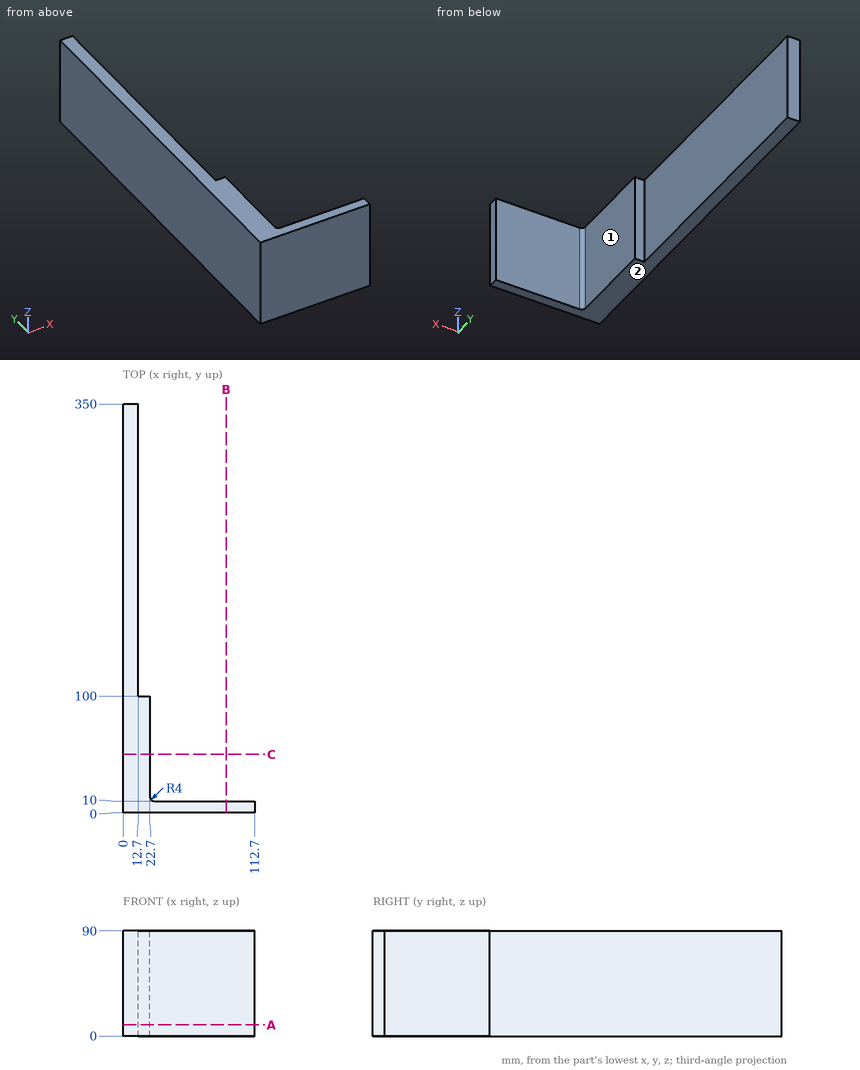
The figure shows three views and two pictorial views of one solid part (mm, origin at its lowest corner). Answer the questions. A direction names the side the tool comes from. Give positions to 0.01 mm unless a question says otherwise; leave off trailing zeros. Order: outer loops, then holes, each group sorted by start corner. A loop starts at its lowest first (then second) coordinate and runs counter-clockwise, first axis right, second up. Notation, with made-up numbers: M 10,-17.5 L 55,-17.5 A9 cw 55,-9.5 Z; hole C 69,27.5 d3. An arc over 180 degrees is marked long. Return JSON: item names as keys, results as strings.
1) Each of these flat-tipped pins is pushed along its axis until it touches: pin 1 (8 mm diameter, centred on x = 55.5, z = 29, fed in from -Y); pin 2 (5 mm diameter, centred on x = 19.5, z = 58, fed in from +Y); pin 3 (2 mm diameter, centred on y = 63, z = 29, fed in from +X). Where does it stop, or does it pass through?
Resolved:
{"pin 1": "y = 0", "pin 2": "y = 100", "pin 3": "x = 22.7"}
2) Section A-A, the plane z = 9.5 is taken. Write down the section's boundary in (x, y), plus the area to 3 significant figures.
Resolved:
{"outline": "M 0,0 L 112.7,0 L 112.7,10 L 26.7,10 A4 cw 22.7,14 L 22.7,100 L 12.7,100 L 12.7,350 L 0,350 Z", "area": "6,350 mm^2"}
3) Straight lines are drawn through the part: line 1 along Y through (x, z) = (82, 58); line 2 along X through (y, z) = (81, 55.5); line 3 along Y through (x, z) = (13.5, 45). For each, find the intervals that lie inside material, in ascending order. Write a range as [from, to].
Resolved:
{"line 1": "[0, 10]", "line 2": "[0, 22.7]", "line 3": "[0, 100]"}
4) Section B-B, the plane x = 88 is taken. Write down the section's boundary in (y, z).
Resolved:
{"outline": "M 0,0 L 10,0 L 10,90 L 0,90 Z"}
5) A tool of negligible diameter and unlimited length cuts with its end or side. For the marked faces 1 and 2, from which of +Z, -Z, +X, -X, +Y, -Y can it reach the whole face along a straight path? Write none if from no direction.
Resolved:
{"face 1": "+Z, -Z, +X, +Y", "face 2": "-Z, +X, -X, +Y, -Y"}
6) Section C-C, the plane y = 50 is taken. Write down the section's boundary in (x, z).
Resolved:
{"outline": "M 0,0 L 22.7,0 L 22.7,90 L 0,90 Z"}
